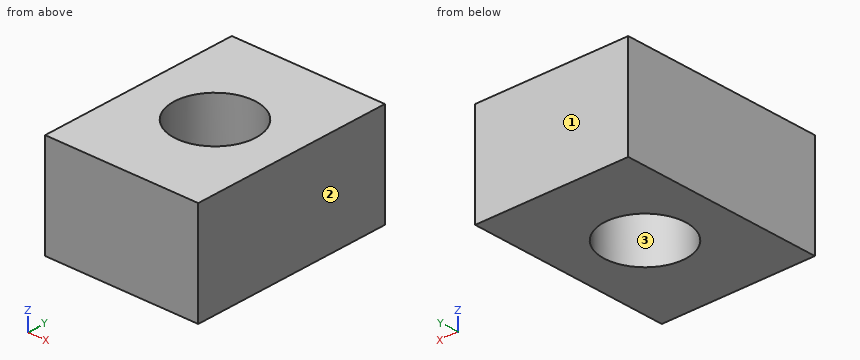
Autodesk Inventor part; units mm, degrees
ref_plane "YZ Plane" through (0, 0, 0) normal (1, 0, 0) x (0, 1, 0)
ref_plane "XZ Plane" through (0, 0, 0) normal (0, 1, 0) x (-1, 0, 0)
ref_plane "XY Plane" through (0, 0, 0) normal (0, 0, 1) x (1, 0, 0)
sketch "Sketch1" plane through (0, 0, 0) normal (0, 0, 1) x (1, 0, 0)
  line L0 (-0.2511, -0.0105) -> (7.2489, -0.0105)
  line L1 (7.2489, -0.0105) -> (7.2489, 9.9895)
  line L2 (7.2489, 9.9895) -> (-0.2511, 9.9895)
  line L3 (-0.2511, 9.9895) -> (-0.2511, -0.0105)
  circle A0 centre (3.4989, 4.9895) radius 2
  point P0 (7.2471, -0.0105)
  dimension "d2" = 4
  dimension "d3" = 5
  dimension "d4" = 7.5
  dimension "d5" = 10
  dimension "d6" = 3.75
extrude "Extrusion1" add sketch "Sketch1" along normal blind 5
properties part number "short back plate spacer" material "ABS Plastic"
Read the model definition and answer for the solid it produces. Units are mm, in the model's axes. Face numbers are marked on the shaded views. Coordinates: 2 decimals unless noted, no trailing zeros. Loops run counter-clockwise (first coordinate to the right, second up) from the corner with the lowest first, then second, coordinate; pieces in that order, holes last. Notation, with made-up numbers: (-26.5, -8.75) -> (-16.5, -8.75) arc R8 cw to (-16.5, -3.75) -> close; hole circle Ø9 at (19.5, 41.25). An arc over 180 degrees is marked (long way). Return JSON: item names as keys, results as strings.
Item 1: For a pull along Y with two mould halves and no side action, classify the marked faces 1, 2 and 3 as +Y half, -Y half, draft (parallel to the pull), parting line (faces both ways), or undercut.
Answers:
{"face 1": "+Y half", "face 2": "draft", "face 3": "undercut"}
Item 2: Find the intervals of material crossed by probe 1 along X at (y, z) = (5, 1.3); probe 2 along Y at (x, z) = (3.5, 3.4); probe 3 along X at (y, z) = (3.75, 1.3), in increasing order.
Answers:
{"probe 1": "x = -0.25 to 1.5, 5.5 to 7.25", "probe 2": "y = -0.01 to 2.99, 6.99 to 9.99", "probe 3": "x = -0.25 to 1.93, 5.07 to 7.25"}
Item 3: Find section C-C (z = 2.15). Determine the outline of the cut face in (x, y), plus the area to 3 significant figures.
Answers:
{"outline": "(-0.25, -0.01) -> (7.25, -0.01) -> (7.25, 9.99) -> (-0.25, 9.99) -> close; hole circle Ø4 at (3.5, 4.99)", "area": "62.4 mm2"}
Item 4: Find section B-B (x = 5). Determine the outline of the cut face in (y, z), plus the area to 3 significant figures.
Answers:
{"outline": "(-0.01, 0) -> (3.67, 0) -> (3.67, 5) -> (-0.01, 5) -> close; (6.31, 0) -> (9.99, 0) -> (9.99, 5) -> (6.31, 5) -> close", "area": "36.8 mm2"}
Item 5: Find section A-A (y = 5.5). Determine the outline of the cut face in (x, z), plus the area to 3 significant figures.
Answers:
{"outline": "(-0.25, 0) -> (1.57, 0) -> (1.57, 5) -> (-0.25, 5) -> close; (5.43, 0) -> (7.25, 0) -> (7.25, 5) -> (5.43, 5) -> close", "area": "18.2 mm2"}
